Verification items for the finished model (mm, model axes). A direction names the side the tool comes from. Round coordinates to 2 decimals unless told otherwise and drop trailing zeros. Order: outer loops, then holes, each group sorted by start corner. A loop starts at its lowest first (then second) coordinate and runs counter-clockwise, first axis right, second up. Notation, with made-up numbers: (-10, 83) -> (48, 83) arc R15 cw to (48, 104) -> close; hole circle Ø1 at (78, 56.5). An arc over 180 degrees is marked (long way). Put each result on its own line as item: value.
Autodesk Inventor part; units mm, degrees
ref_plane "YZ Plane" through (0, 0, 0) normal (1, 0, 0) x (0, 1, 0)
ref_plane "XZ Plane" through (0, 0, 0) normal (0, 1, 0) x (-1, 0, 0)
ref_plane "XY Plane" through (0, 0, 0) normal (0, 0, 1) x (1, 0, 0)
sketch "Эскиз1" plane through (0, 0, 0) normal (0, 1, 0) x (-1, 0, 0)
  line L0 (0, 0) -> (-7, 0) construction
  line L1 (0, 4) -> (-7, 4)
  line L2 (-7, -4) -> (0, -4)
  arc A0 (0, -4) -> (0, 4) centre (0, 0) ccw
  arc A1 (-7, 4) -> (-7, -4) centre (-7, 0) ccw
  point P0 (-3.5, 0)
  dimension "d0" = 7
  dimension "d1" = 8
extrude "Выдавливание1" add sketch "Эскиз1" along normal blind 5
sketch "Эскиз2" plane through (0, 0, 0) normal (0, -1, 0) x (1, 0, 0)
  line L0 (0, 4) -> (7, 4)
  arc A0 (0, 4) -> (0, -4) centre (0, 0) ccw
  line L1 (7, -4) -> (0, -4)
  arc A1 (7, -4) -> (7, 4) centre (7, 0) ccw
  arc A2 (0, 6) -> (0, -6) centre (0, 0) ccw
  line L2 (0, 6) -> (7, 6)
  arc A3 (7, -6) -> (7, 6) centre (7, 0) ccw
  line L3 (7, -6) -> (0, -6)
  dimension "d4" = 2
extrude "Выдавливание2" add sketch "Эскиз2" against normal blind 1
sketch "Эскиз3" plane through (0, 5, 0) normal (0, 1, 0) x (1, 0, 0)
  line L0 (0, -4) -> (7, -4)
  arc A0 (7, -4) -> (7, 4) centre (7, 0) ccw
  line L1 (7, 4) -> (0, 4)
  arc A1 (0, 4) -> (0, -4) centre (0, 0) ccw
  line L2 (0, 3) -> (7, 3)
  arc A2 (7, -3) -> (7, 3) centre (7, 0) ccw
  line L3 (7, -3) -> (0, -3)
  arc A3 (0, 3) -> (0, -3) centre (0, 0) ccw
  dimension "d7" = 1
extrude "Выдавливание3" cut sketch "Эскиз3" against normal up to surface (5 mm away) contours L2 A2 L3 A3
properties part number "Flanec_podProvoda"
Item 1: Section check A-A on x = 2.5. Record the boundary of the cut face in (y, z), then the cut area to 3 significant figures.
Check sheet entries:
outline: (0, -6) -> (1, -6) -> (1, -4) -> (5, -4) -> (5, -3) -> (0, -3) -> close; (0, 3) -> (5, 3) -> (5, 4) -> (1, 4) -> (1, 6) -> (0, 6) -> close
area: 14.0 mm^2
Item 2: Tool access check on faces 1 (the flat face through (3, 1, 5)), 2 (the cylindrical face through (-4, 3, 0)), 3 (the cylindrical face through (-3, 3, 0)). Record the directions out of +Z, -Z, +X, -X, +Y, -Y that give a thin tool (end or side, any length) a straight path to the whole face; none if there is none.
Check sheet entries:
face 1: +Y
face 2: -X, +Y
face 3: +Y, -Y
Item 3: Material ranges on L1, parallel to Z at x = 4, y = 4.4; L2, parallel to Y at x = 9.5, z = 4; L3, parallel to Z at x = 8, y = 2.4, recorded low to high. Write a range as [from, to].
Check sheet entries:
L1: z = [-4, -3], [3, 4]
L2: y = [0, 1]
L3: z = [-3.87, -2.83], [2.83, 3.87]
Item 4: Release check for a two-part mould opening along Z. For faces 4 (the flat face through (3, 0, -4)), 5 (the cylindrical face through (13, 0.5, -0.1)), 6 (the cylindrical face through (10, 3, 0)) record: +Z half, -Z half, draft (parallel to the pull), parting line (faces both ways), or undercut.
Check sheet entries:
face 4: draft
face 5: parting line
face 6: undercut
Item 5: Section check C-C on y = 4.15. Record the boundary of the cut face in (x, z).
Check sheet entries:
outline: (0, -4) -> (7, -4) arc R4 ccw to (7, 4) -> (0, 4) arc R4 ccw to start; hole (0, -3) -> (7, -3) arc R3 ccw to (7, 3) -> (0, 3) arc R3 ccw to start
Item 6: Section check B-B on z = 0. Record the boundary of the cut face in (x, y).
Check sheet entries:
outline: (-6, 0) -> (-3, 0) -> (-3, 5) -> (-4, 5) -> (-4, 1) -> (-6, 1) -> close; (10, 0) -> (13, 0) -> (13, 1) -> (11, 1) -> (11, 5) -> (10, 5) -> close
Item 7: Gauge pin test, flat ends, axial feed: pin 1 Ø3 at (x, z) = (-3.5, 4.5) entering from -Y; pin 2 Ø1.5 at (y, z) = (1.5, 3) entering from +X; pin 3 Ø1.2 at (x, y) = (4.5, 3) entering from +Z; pin 4 Ø3 at (y, z) = (4, -2.5) entering from +X. Record the tip position at first contact, or that the pin passes through.
Check sheet entries:
pin 1: stops at y = 0
pin 2: stops at x = 12.48
pin 3: stops at z = 4
pin 4: stops at x = 10.87
Item 8: Section check D-D on z = 4.5. Record the boundary of the cut face in (x, y).
Check sheet entries:
outline: (-3.97, 0) -> (10.97, 0) -> (10.97, 1) -> (-3.97, 1) -> close
